Here's how the part is built. I have some questions about the finished solid (model axes, mm). A direction names the side the tool comes from. Round coordinates to 2 decimals unless told otherwise and drop trailing zeros. Order: outer loops, then holes, each group sorted by start corner. A loop starts at its lowest first (then second) coordinate and runs counter-clockwise, first axis right, second up.
```python
from build123d import *

# Parameters (mm, degrees)
F0_W     = 25
F0_H     = 25
F1_DEPTH = 3


with BuildPart() as f1:
    # F0 (on Top) → F1 (new body)
    with BuildSketch(Plane.XY):
        with BuildLine():
            ThreePointArc((27.5, 27.5), (0, 20.826823), (-27.5, 27.5))
            ThreePointArc((-27.5, 27.5), (-23.195683, 0), (-27.5, -27.5))
            ThreePointArc((-27.5, -27.5), (0, -24.772539), (27.5, -27.5))
            ThreePointArc((27.5, -27.5), (26.236924, 0), (27.5, 27.5))
        make_face()
        Rectangle(F0_W, F0_H, mode=Mode.SUBTRACT)
    extrude(amount=F1_DEPTH)


solid = f1.part
```
1. If we section it at B-B, the plane y = -6: Write out the boundary of the cut face in (x, z), and give its area (3 significant figures).
Evaluation:
outline: (-23.4, 0) - (-12.5, 0) - (-12.5, 3) - (-23.4, 3) - close; (12.5, 0) - (26.3, 0) - (26.3, 3) - (12.5, 3) - close
area: 74.1 mm2
2. On a 3-axis mill with a long thin cutter (end or side, diameter ignored), from which of +Z, -Z, +X, -X, +Y, -Y can I reach the whole of each face in a straight line? I mean faces 1 (the flat face through (0, 12.5, 1)), 2 (the cylindrical face through (-23.197, 0.391, 1.479)). Say none if no direction works.
Evaluation:
face 1: +Z, -Z
face 2: +Z, -Z, -X
3. I'm going to push flat-ended pins straight in: P1, Ø1.5, axis at x = -15.5, y = -3.5, coming from the -Z side; P2, Ø1.5, axis at x = 6, z = 1, coming from the -Y side; P3, Ø1.5, axis at y = -2, z = 1, coming from the -X side; P4, Ø1, axis at x = 7, z = 2.5, coming from the +Y side. Where does each tip first touch, or does it pass through?
Evaluation:
P1: stops at z = 0
P2: stops at y = -24.94
P3: stops at x = -23.24
P4: stops at y = 21.3
4. I need wall thicknesses on probe 1 along Y at (x, z) = (0.5, 2.6); probe 2 along X at (y, z) = (6, 0.85); probe 3 along Y at (x, z) = (5, 0.5). Which ranges of each line are inside material? Lowest first, please.
Evaluation:
probe 1: y = -24.77 to -12.5, 12.5 to 20.83
probe 2: x = -23.4 to -12.5, 12.5 to 26.3
probe 3: y = -24.86 to -12.5, 12.5 to 21.04
5. If we section it at D-D, the plane x = -16.5: Write out the boundary of the cut face in (y, z).
Evaluation:
outline: (-25.75, 0) - (23.14, 0) - (23.14, 3) - (-25.75, 3) - close
6. If we section it at A-A, the plane z = 1.3: Write out the boundary of the cut face in (x, y).
Evaluation:
outline: (-27.5, -27.5) arc R140 cw to (27.5, -27.5) arc R300 cw to (27.5, 27.5) arc R60 cw to (-27.5, 27.5) arc R90 cw to start; hole (-12.5, -12.5) - (12.5, -12.5) - (12.5, 12.5) - (-12.5, 12.5) - close
7. If we section it at C-C, the plane x = -8.5: Write out the boundary of the cut face in (y, z), and give its area (3 significant figures).
Evaluation:
outline: (-25.03, 0) - (-12.5, 0) - (-12.5, 3) - (-25.03, 3) - close; (12.5, 0) - (21.43, 0) - (21.43, 3) - (12.5, 3) - close
area: 64.4 mm2
8. If we mould it in two halves opening along Y, with no side actions, what happens to faces 3 (the flat face through (0, -12.5, 1)), 4 (the cylindrical face through (26.237, -0.386, 1.479)), 5 (the cylindrical face through (-0.388, -24.773, 1.479)), 6 (the flat face through (-13, 0, 0))? For each: released by +Y, released by -Y, zero draft, split by the parting line, or undercut.
Evaluation:
face 3: undercut
face 4: undercut
face 5: released by -Y
face 6: zero draft
